```python
from build123d import *

# Parameters (mm, degrees)
BASE_EXTRUDE_DEPTH = 101.6
SLOT_DEPTH         = 112.588942245
LPATTERN1_COUNT    = 2
LPATTERN1_PITCH    = 50.8


with BuildPart() as part:
    # Sketch1 → Base-Extrude (new body)
    with BuildSketch(Plane.XY):
        with BuildLine():
            Line((-11.3109375, 20.6375), (-18.8515625, 20.6375))
            ThreePointArc((-18.8515625, 20.6375), (-20.114411017, 20.114411017), (-20.6375, 18.8515625))
            Line((-20.6375, 18.8515625), (-20.6375, -18.8515625))
            ThreePointArc((-20.6375, -18.8515625), (-20.114411017, -20.114411017), (-18.8515625, -20.6375))
            Line((-18.8515625, -20.6375), (18.8515625, -20.6375))
            ThreePointArc((18.8515625, -20.6375), (20.114411017, -20.114411017), (20.6375, -18.8515625))
            Line((20.6375, -18.8515625), (20.6375, 18.8515625))
            ThreePointArc((20.6375, 18.8515625), (20.114411017, 20.114411017), (18.8515625, 20.6375))
            Line((18.8515625, 20.6375), (11.3109375, 20.6375))
            ThreePointArc((11.3109375, 20.6375), (10.048088983, 20.114411017), (9.525, 18.8515625))
            Line((9.525, 18.8515625), (9.525, 13.49375))
            Line((9.525, 13.49375), (13.096875, 13.49375))
            Line((13.096875, 13.49375), (13.096875, 17.065625))
            Line((13.096875, 17.065625), (17.065625, 17.065625))
            Line((17.065625, 17.065625), (17.065625, -17.065625))
            Line((17.065625, -17.065625), (-17.065625, -17.065625))
            Line((-17.065625, -17.065625), (-17.065625, 17.065625))
            Line((-17.065625, 17.065625), (-13.096875, 17.065625))
            Line((-13.096875, 17.065625), (-13.096875, 13.49375))
            Line((-13.096875, 13.49375), (-9.525, 13.49375))
            Line((-9.525, 13.49375), (-9.525, 18.8515625))
            ThreePointArc((-9.525, 18.8515625), (-10.048088983, 20.114411017), (-11.3109375, 20.6375))
        make_face()
    extrude(amount=BASE_EXTRUDE_DEPTH)

    # Sketch2 → Slot (cut, through all)
    with BuildSketch(Plane.XZ.offset(20.6375)):
        with BuildLine():
            Line((7.14375, 32.54375), (7.14375, 18.25625))
            ThreePointArc((7.14375, 18.25625), (0, 11.1125), (-7.14375, 18.25625))
            Line((-7.14375, 18.25625), (-7.14375, 32.54375))
            ThreePointArc((-7.14375, 32.54375), (0, 39.6875), (7.14375, 32.54375))
        make_face()
    slot = extrude(amount=-SLOT_DEPTH, mode=Mode.SUBTRACT)

    # LPattern1: Slot ×2
    with Locations(*[(0, 0, i * LPATTERN1_PITCH) for i in range(1, LPATTERN1_COUNT)]):
        add(slot, mode=Mode.SUBTRACT)


solid = part.part
```
Work out the finished part from the listing and answer in its coordinate system (mm). A direction names the side the tool comes from. Give positions to 0.01 mm unless a question says otherwise; leave off trailing zeros. Order: outer loops, then holes, each group sorted by start corner. A loop starts at its lowest first (then second) coordinate and runs counter-clockwise, first axis right, second up. Notation, with made-up numbers: (-0.75, 2.25) -> (54.25, 2.25) arc R18 ccw to (54.25, 27.25) -> close; hole circle Ø9 at (45, 45). An arc over 180 degrees is marked (long way). Answer as CSV lines item,"result". Start each with the question number.
(1) Consider line 1 along X through (y, z) = (15, 31) (1 decimal); line 2 along X through (y, z) = (7, 36). Determine where each line is inside the solid, lowest interval first.
(2) Section C-C, the plane x = -15 is taken. Write down the section's boundary in (y, z).
(3) Section A-A, the plane y = 16 is taken. Write down the section's boundary in (x, z) (1 decimal), plus the area to 3 significant figures.
(4) For a pull along Y with two mould halves and no side action, classify faces 6 (the cylindrical face through (10.062, 20.128, 50.089)), 7 (the flat face through (17.066, 0, 50)), 8 (the cylindrical face through (0.157, -18.877, 11.114)) as released by +Y, released by -Y, zero draft, split by the parting line, or undercut.
(5) Section B-B, the plane z = 72.5 is taken. Write down the section's boundary in (x, y) (1 decimal), plus the area to 3 significant figures.
(6) Each of these flat-tipped pins is pushed along its axis until it touches: pin 1 Ø1.1 at (y, z) = (-19.5, 26) entering from +X; pin 2 Ø17 at (x, z) = (-0.5, 38) entering from +Y. Where does it stop, or does it pass through?
(7) Which of the six approach directions +Z, -Z, +X, -X, +Y, -Y give full straight-line access (tool end or side, diameter ignored) to faces 1 (the cylindrical face through (-20.1, 20.13, 50.09)), 2 (the flat face through (0, -18, 0)), 3 (the cylindrical face through (-0.157, -18.877, 90.486)), 4 (the flat face through (-13.097, 15, 50)), 5 (the cylindrical face through (-10.034, 20.1, 50.089))?
Entries:
1,line 1,"-20.6 to -17.1, -13.1 to -9.5, 9.5 to 13.1, 17.1 to 20.6"
1,line 2,"-20.64 to -17.07, 17.07 to 20.64"
2,outline,"(-20.64, 0) -> (-17.07, 0) -> (-17.07, 101.6) -> (-20.64, 101.6) -> close; (17.07, 0) -> (20.64, 0) -> (20.64, 101.6) -> (17.07, 101.6) -> close"
3,outline,"(-20.6, 0) -> (-17.1, 0) -> (-17.1, 101.6) -> (-20.6, 101.6) -> close; (-13.1, 0) -> (-9.5, 0) -> (-9.5, 101.6) -> (-13.1, 101.6) -> close; (9.5, 0) -> (13.1, 0) -> (13.1, 101.6) -> (9.5, 101.6) -> close; (17.1, 0) -> (20.6, 0) -> (20.6, 101.6) -> (17.1, 101.6) -> close"
3,area,"1,450 mm²"
4,face 6,"released by +Y"
4,face 7,"undercut"
4,face 8,"zero draft"
5,outline,"(-20.6, -18.9) arc R1.8 ccw to (-18.9, -20.6) -> (-7.1, -20.6) -> (-7.1, -17.1) -> (-17.1, -17.1) -> (-17.1, 17.1) -> (-13.1, 17.1) -> (-13.1, 13.5) -> (-9.5, 13.5) -> (-9.5, 18.9) arc R1.8 ccw to (-11.3, 20.6) -> (-18.9, 20.6) arc R1.8 ccw to (-20.6, 18.9) -> close; (7.1, -20.6) -> (18.9, -20.6) arc R1.8 ccw to (20.6, -18.9) -> (20.6, 18.9) arc R1.8 ccw to (18.9, 20.6) -> (11.3, 20.6) arc R1.8 ccw to (9.5, 18.9) -> (9.5, 13.5) -> (13.1, 13.5) -> (13.1, 17.1) -> (17.1, 17.1) -> (17.1, -17.1) -> (7.1, -17.1) -> close"
5,area,"441 mm²"
6,pin 1,"x = 20.63"
6,pin 2,"y = -17.07"
7,face 1,"+Z, -Z, -X, +Y"
7,face 2,"-Z, +X, -X, +Y, -Y"
7,face 3,"+Y, -Y"
7,face 4,"+Z, -Z"
7,face 5,"+Z, -Z, +Y"
